```python
from build123d import *

# Parameters (mm, degrees)
SKETCH_W        = 29
SKETCH_H        = 47
PAD_DEPTH       = 40
SKETCH001_R     = 9.75
PAD001_DEPTH    = 10
SKETCH002_W     = 56
SKETCH002_H     = 6
POCKET_DEPTH    = 100
POCKET001_DEPTH = 5
SKETCH005_R     = 0.9
POCKET002_DEPTH = 5
SKETCH006_W     = 40
SKETCH006_H     = 20
PAD002_DEPTH    = 10
SKETCH007_R     = 3
HOLE_DEPTH      = 50
SKETCH008_W     = 40
SKETCH008_H     = 45
POCKET003_DEPTH = 68.991653
SKETCH009_W     = 40
SKETCH009_H     = 5
PAD003_DEPTH    = 50
SKETCH010_W     = 40
SKETCH010_H     = 70
PAD004_DEPTH    = 45


with BuildPart() as part:
    # Sketch → Pad (new body)
    with BuildSketch(Plane.XY.offset(10)):
        with BuildLine():
            Line((0, 0), (40, 0))
            Line((40, 0), (40, 60))
            ThreePointArc((40, 60), (20, 68.990653), (0, 60))
            Line((0, 60), (0, 0))
        make_face()
        with Locations((20, 30)):
            Rectangle(SKETCH_W, SKETCH_H, mode=Mode.SUBTRACT)
    extrude(amount=PAD_DEPTH)

    # Sketch001 (on Face9 of Pad) → Pad001 (join)
    with BuildSketch(Plane(origin=(0, 0, 10), x_dir=(1, 0, 0), z_dir=(0, 0, -1))):
        with BuildLine():
            Line((40, -60), (40, 30))
            ThreePointArc((40, 30), (20, 50), (0, 30))
            Line((0, 30), (0, -60))
            ThreePointArc((0, -60), (20, -68.990653), (40, -60))
        make_face()
        with Locations((20, -42.25)):
            Circle(SKETCH001_R, mode=Mode.SUBTRACT)
    extrude(amount=PAD001_DEPTH)

    # Sketch002 (on Face7 of Pad001) → Pocket (cut)
    with BuildSketch(Plane(origin=(0, 0, 0), x_dir=(0, -1, 0), z_dir=(-1, 0, 0))):
        with Locations((-48, 3)):
            Rectangle(SKETCH002_W, SKETCH002_H)
    extrude(amount=-POCKET_DEPTH, mode=Mode.SUBTRACT)

    # Sketch003 (on Face4 of Pocket) → Pocket001 (cut)
    with BuildSketch(Plane.XY.offset(10)):
        with BuildLine():
            Line((0, 0), (40, 0))
            Line((40, 0), (40, -30))
            ThreePointArc((0, -30), (20, -50), (40, -30))
            Line((0, -30), (0, 0))
        make_face()
    extrude(amount=-POCKET001_DEPTH, mode=Mode.SUBTRACT)

    # Sketch005 → Pocket002 (cut)
    with BuildSketch(Plane(origin=(0, 0, 0), x_dir=(1, 0, 0), z_dir=(0, 0, -1))):
        with Locations((11.98, 30)):
            Circle(SKETCH005_R)
        with Locations((14.34, 35.7)):
            Circle(SKETCH005_R)
        with Locations((20, 37.98)):
            Circle(SKETCH005_R)
        with Locations((25.66, 35.7)):
            Circle(SKETCH005_R)
        with Locations((28.02, 30)):
            Circle(SKETCH005_R)
        with Locations((25.66, 24.35)):
            Circle(SKETCH005_R)
        with Locations((20, 22.02)):
            Circle(SKETCH005_R)
        with Locations((14.34, 24.34)):
            Circle(SKETCH005_R)
    extrude(amount=-POCKET002_DEPTH, mode=Mode.SUBTRACT)

    # Sketch006 (on Face17 of Pocket002) → Pad002 (join)
    with BuildSketch(Plane(origin=(0, 0, 0), x_dir=(1, 0, 0), z_dir=(0, 0, -1))):
        with Locations((20, -10)):
            Rectangle(SKETCH006_W, SKETCH006_H)
    extrude(amount=PAD002_DEPTH)

    # Sketch007 → Hole (cut)
    with BuildSketch(Plane.YZ.offset(40)):
        with Locations((10, -5)):
            Circle(SKETCH007_R)
    extrude(amount=-HOLE_DEPTH, mode=Mode.SUBTRACT)

    # Sketch008 (on Face1 of Hole) → Pocket003 (cut, through all)
    with BuildSketch(Plane.XZ):
        with Locations((20, 27.5)):
            Rectangle(SKETCH008_W, SKETCH008_H)
    extrude(amount=-POCKET003_DEPTH, mode=Mode.SUBTRACT)

    # Sketch009 (on Face14 of Pocket003) → Pad003 (join)
    with BuildSketch(Plane(origin=(0, 20, 0), x_dir=(-1, 0, 0), z_dir=(0, 1, 0))):
        with Locations((-20, 2.5)):
            Rectangle(SKETCH009_W, SKETCH009_H)
    extrude(amount=PAD003_DEPTH)

    # Sketch010 (on Face2 of Pad003) → Pad004 (join)
    with BuildSketch(Plane.XY.offset(5)):
        with Locations((20, 35)):
            Rectangle(SKETCH010_W, SKETCH010_H)
    extrude(amount=PAD004_DEPTH)


solid = part.part
```
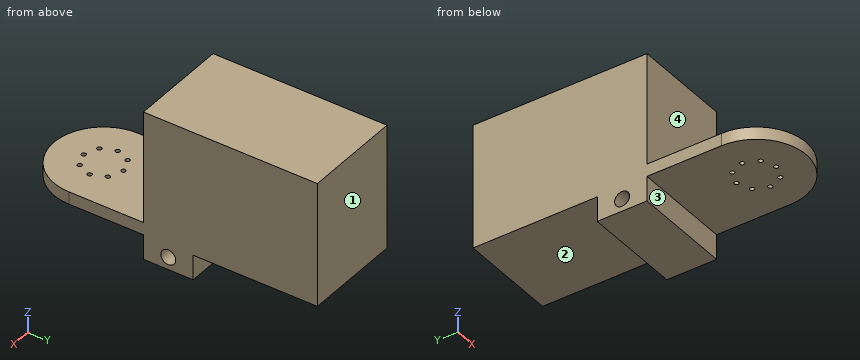
Geometry check sheet. Reference: the model listing, model coordinates, mm. Face numbers are marked on the shaded views. A direction names the side the tool comes from. Coordinates: 2 decimals unless noted, no trailing zeros. Write each loop counter-clockwise with the first axis right and the second up, starting at its lowest first coordinate (ties: lowest second). Pieces come first, ordered by that corner, then holes. Notation, with made-up numbers: M 83,72 L 100,72 A22 ccw 100,96 Z; hole C -19.5,4 d10. An arc over 180 degrees is marked long. Answer as a JSON object with one key per item and string values.
1. Section check D-D, the plane y = 48. Enter the section's corners in (x, z), plus the area to 3 significant figures.
Answers below:
{"outline": "M 0,0 L 40,0 L 40,50 L 0,50 Z", "area": "2,000 mm²"}
2. Scan lines: L1, parallel to X at y = -24, z = 3; L2, parallel to X at y = -22, z = 1; L3, parallel to Y at x = 14.34, z = 2.1. Record each from-to range of solid material in increasing order.
Answers below:
{"L1": "x = 0 to 13.51, 15.17 to 24.83, 26.49 to 40", "L2": "x = 0 to 19.1, 20.9 to 40", "L3": "y = -49.18 to -36.6, -34.8 to -25.24, -23.44 to 70"}
3. Go/stop test with flat-tipped pins: pin 1 Ø12 at (x, y) = (26, 52.5) entering from -Z; pin 2 Ø12 at (x, y) = (15.5, -28) entering from +Z; pin 3 Ø1.1 at (x, y) = (28.02, -30) entering from -Z; pin 4 Ø11 at (x, z) = (21.5, -6) entering from -Y. Record where each tip stops, or that it passes through.
Answers below:
{"pin 1": "stops at z = 0", "pin 2": "stops at z = 5", "pin 3": "passes through", "pin 4": "stops at y = 0"}
4. Section check A-A, the plane y = 10. Enter the section's corners in (x, z), plus the area to 3 significant figures.
Answers below:
{"outline": "M 0,-10 L 40,-10 L 40,-8 L 0,-8 Z; M 0,-2 L 40,-2 L 40,50 L 0,50 Z", "area": "2,160 mm²"}
5. Tool access check on the marked faces 1, 2, 3 and 4. Record the directions out of +Z, -Z, +X, -X, +Y, -Y that give a thin tool (end or side, any length) a straight path to the whole face; none if there is none.
Answers below:
{"face 1": "+Z, -Z, +X, -X, +Y", "face 2": "-Z, +X, -X, +Y", "face 3": "-Z, +X, -X, -Y", "face 4": "+Z, +X, -X, -Y"}
6. Section check C-C, the plane x = 5. Enter the section's corners in (y, z).
Answers below:
{"outline": "M -43.23,0 L 0,0 L 0,-10 L 20,-10 L 20,0 L 70,0 L 70,50 L 0,50 L 0,5 L -43.23,5 Z; hole C 10,-5 d6"}
7. Section check B-B, the plane z = -5. Enter the section's corners in (x, y), plus the area to 3 significant figures.
Answers below:
{"outline": "M 0,0 L 40,0 L 40,7 L 0,7 Z; M 0,13 L 40,13 L 40,20 L 0,20 Z", "area": "560 mm²"}
